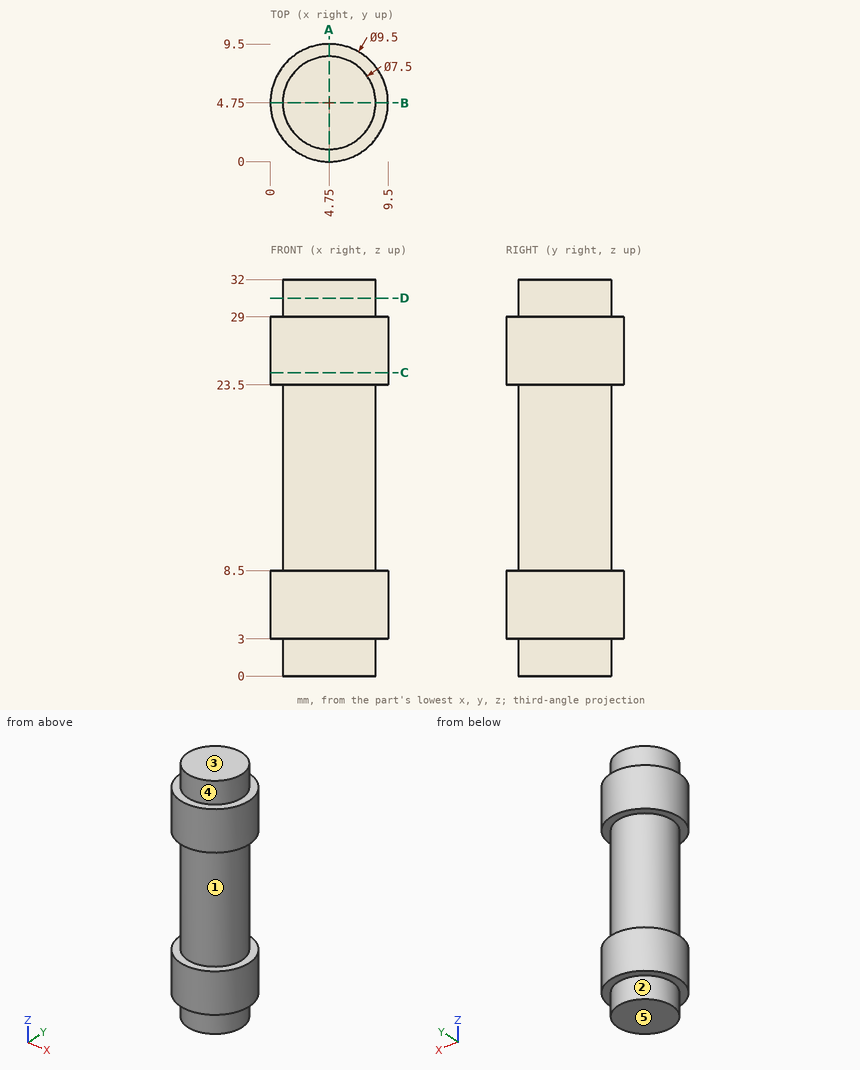
Here's the drawing with two shaded views (mm, measured from the low corner). I have some questions. A direction names the side the tool comes from. Round coordinates to 2 decimals unless told otherwise and drop trailing zeros. Write each loop counter-clockwise with the first axis right and the second up, starting at its lowest first coordinate (ties: lowest second). Pieces come first, ordered by that corner, then holes. Notation, with made-up numbers: M -24.5,54.5 L -20.5,54.5 A26 cw -20.5,89.5 Z; hole C 0,-10 d11. An arc over 180 degrees is marked long. Write each question's results on one line, items separated by ' | '. Start each with the question number.
1. Thinking about a two-plate mould opening in Z: for the marked faces 1, 2 and 3, which applies, +Z half, -Z half, draft (parallel to the pull), parting line (faces both ways), or undercut?
2. On a 3-axis mill with a long thin cutter (end or side, diameter ignored), from which of +Z, -Z, +X, -X, +Y, -Y can I reach the whole of each face in a straight line? I mean the marked faces 4 and 5. Say none if no direction works.
3. I need wall thicknesses on L1, parallel to Z at x = 1, y = 2.5; L2, parallel to Y at x = 4.5, z = 19; L3, parallel to Y at x = 7.5, z = 9.5. Which ranges of each line are inside material? Lowest first, please. Write a range as from..to.
4. I'm going to push a flat-ended pin straight in: pin 1 Ø3 at (y, z) = (6.5, 24.5) entering from +X. Where does the tip first touch, or does it pass through?
5. Imagine slicing it at A-A on x = 4.75. List the corners of the cut face in (y, z) for me, and give its area (3 significant figures).
6. Imagine slicing it at D-D on z = 30.5. List the corners of the cut face in (x, y) for me.
7. Imagine slicing it at C-C on z = 24.5. List the corners of the cut face in (x, y) for me, and give its area (3 significant figures).
Result sheet:
1) face 1: undercut | face 2: draft | face 3: +Z half
2) face 4: +Z | face 5: -Z, +X, -X, +Y, -Y
3) L1: z = 3..8.5, 23.5..29 | L2: y = 1.01..8.49 | L3: y = 2.2..7.3
4) pin 1: stops at x = 9.49
5) outline: M 0,3 L 1,3 L 1,0 L 8.5,0 L 8.5,3 L 9.5,3 L 9.5,8.5 L 8.5,8.5 L 8.5,23.5 L 9.5,23.5 L 9.5,29 L 8.5,29 L 8.5,32 L 1,32 L 1,29 L 0,29 L 0,23.5 L 1,23.5 L 1,8.5 L 0,8.5 Z | area: 262 mm^2
6) outline: C 4.75,4.75 d7.5
7) outline: C 4.75,4.75 d9.5 | area: 70.9 mm^2
